Check sheet for the modelled part. Datum: model origin and axes. Units: mm. A direction names the side the tool comes from. Give positions to 0.01 mm unless a question says otherwise; leave off trailing zeros. Order: outer loops, then holes, each group sorted by start corner. A loop starts at its lowest first (then second) coordinate and runs counter-clockwise, first axis right, second up.
from build123d import *

# Parameters (mm, degrees)
SKETCH1_W           = 68
SKETCH1_H           = 68
BOSS_EXTRUDE1_DEPTH = 41
CUT_EXTRUDE1_START  = 41
SKETCH2_W           = 64
SKETCH2_H           = 64
CUT_EXTRUDE1_DEPTH  = 32
CUT_EXTRUDE4_START  = 9
SKETCH3_R           = 23
CUT_EXTRUDE4_DEPTH  = 2
CUT_EXTRUDE9_START  = 7
SKETCH5_R           = 6.05
CUT_EXTRUDE9_DEPTH  = 8
SKETCH6_R           = 10.5
CUT_EXTRUDE10_DEPTH = 5
SKETCH7_W           = 30
SKETCH7_H           = 30
SKETCH7_W_2         = 26
SKETCH7_H_2         = 26
CUT_EXTRUDE11_DEPTH = 2
SKETCH8_R           = 1.5
CUT_EXTRUDE12_DEPTH = 3
SKETCH4_W           = 11
SKETCH4_H           = 16
SKETCH4_R           = 1.75
CUT_EXTRUDE13_DEPTH = 3


with BuildPart() as part:
    # Sketch1 → Boss-Extrude1 (new body)
    with BuildSketch(Plane(origin=(0, 0, 0), x_dir=(1, 0, 0), z_dir=(0, 1, 0))):
        Rectangle(SKETCH1_W, SKETCH1_H)
    extrude(amount=BOSS_EXTRUDE1_DEPTH)

    # Sketch2 → Cut-Extrude1 (cut)
    with BuildSketch(Plane(origin=(0, 0, 0), x_dir=(1, 0, 0), z_dir=(0, 1, 0)).offset(CUT_EXTRUDE1_START)):
        Rectangle(SKETCH2_W, SKETCH2_H)
    extrude(amount=-CUT_EXTRUDE1_DEPTH, mode=Mode.SUBTRACT)

    # Sketch3 → Cut-Extrude4 (cut)
    with BuildSketch(Plane(origin=(0, 0, 0), x_dir=(1, 0, 0), z_dir=(0, 1, 0)).offset(CUT_EXTRUDE4_START)):
        Circle(SKETCH3_R)
    extrude(amount=-CUT_EXTRUDE4_DEPTH, mode=Mode.SUBTRACT)

    # Sketch5 → Cut-Extrude9 (cut, through all)
    with BuildSketch(Plane(origin=(0, 0, 0), x_dir=(1, 0, 0), z_dir=(0, 1, 0)).offset(CUT_EXTRUDE9_START)):
        Circle(SKETCH5_R)
    extrude(amount=-CUT_EXTRUDE9_DEPTH, mode=Mode.SUBTRACT)

    # Sketch6 → Cut-Extrude10 (cut)
    with BuildSketch(Plane.XZ):
        Circle(SKETCH6_R)
    extrude(amount=-CUT_EXTRUDE10_DEPTH, mode=Mode.SUBTRACT)

    # Sketch7 → Cut-Extrude11 (cut)
    with BuildSketch(Plane(origin=(0, 0, 0), x_dir=(-1, 0, 0), z_dir=(0, -1, 0))):
        Rectangle(SKETCH7_W, SKETCH7_H)
        Rectangle(SKETCH7_W_2, SKETCH7_H_2, mode=Mode.SUBTRACT)
    extrude(amount=-CUT_EXTRUDE11_DEPTH, mode=Mode.SUBTRACT)

    # Sketch8 → Cut-Extrude12 (cut, through all)
    with BuildSketch(Plane.ZY.offset(-32)):
        with Locations((-20, 32)):
            Circle(SKETCH8_R)
    extrude(amount=-CUT_EXTRUDE12_DEPTH, mode=Mode.SUBTRACT)

    # Sketch4 → Cut-Extrude13 (cut)
    with BuildSketch(Plane(origin=(0, 7, 0), x_dir=(1, 0, 0), z_dir=(0, 1, 0))):
        with Locations((-18.125903529, 0.086164087)):
            Rectangle(SKETCH4_W, SKETCH4_H)
        with Locations((-16.625903529, 0.086164087)):
            Circle(SKETCH4_R, mode=Mode.SUBTRACT)
    extrude(amount=-CUT_EXTRUDE13_DEPTH, mode=Mode.SUBTRACT)


solid = part.part
1) Section check C-C, the plane y = 32. Record the cut outline in (x, z).
Recorded:
outline: (-34, -34) - (34, -34) - (34, -21.5) - (32, -21.5) - (32, -32) - (-32, -32) - (-32, 32) - (32, 32) - (32, -18.5) - (34, -18.5) - (34, 34) - (-34, 34) - close
2) Depth check by flat-ended pin: pin 1 Ø1.7 at (x, z) = (-22, 3) entering from -Y; pin 2 Ø9 at (x, z) = (-17.5, -2) entering from +Y. Enter the tip coordinate at first touch or a pass-through.
Recorded:
pin 1: stops at y = 0
pin 2: stops at y = 7
3) Draft check along Y on faces 5 (the face through (-18, 6, -8.086)), 6 (the face through (-16, 0, 0)), 7 (the face through (-15, 1, 0)). Enter one of: +Y half, -Y half, draft (parallel to the pull), parting line (faces both ways), or undercut.
Recorded:
face 5: undercut
face 6: -Y half
face 7: draft
4) Section check D-D, the plane x = 29. Record the cut outline in (y, z), then the cut area to 3 significant figures.
Recorded:
outline: (0, -34) - (41, -34) - (41, -32) - (9, -32) - (9, 32) - (41, 32) - (41, 34) - (0, 34) - close
area: 740 mm2
5) Material ranges on L1, parallel to X at y = 5.6, z = 0; L2, parallel to Z at x = 0, y = 1; L3, parallel to X at y = 12, z = -6.5, recorded low to high.
Recorded:
L1: x = -34 to -23.63, -18.37 to -14.88, -12.63 to -6.05, 6.05 to 34
L2: z = -34 to -15, -13 to -10.5, 10.5 to 13, 15 to 34
L3: x = -34 to -32, 32 to 34
6) Section check A-A, the plane x = 0. Record the cut outline in (y, z), then the cut area to 3 significant figures.
Recorded:
outline: (0, -34) - (41, -34) - (41, -32) - (9, -32) - (9, -23) - (7, -23) - (7, -6.05) - (5, -6.05) - (5, -10.5) - (0, -10.5) - (0, -13) - (2, -13) - (2, -15) - (0, -15) - close; (0, 10.5) - (5, 10.5) - (5, 6.05) - (7, 6.05) - (7, 23) - (9, 23) - (9, 32) - (41, 32) - (41, 34) - (0, 34) - (0, 15) - (2, 15) - (2, 13) - (0, 13) - close
area: 511 mm2
7) Set-up check for faces 1 (the face through (-18, 6, 7.914)), 2 (the face through (32.99, 32.07, -21.5)), 3 (the face through (5, 7, 5)), 4 (the face through (13, 1, 0)): record each of +Z, -Z, +X, -X, +Y, -Y from which the full face is reachable in a straight line by a thin tool's end or side.
Recorded:
face 1: none
face 2: +X
face 3: +Y
face 4: -Y
8) Section check B-B, the plane z = 26. Record the cut outline in (x, y).
Recorded:
outline: (-34, 0) - (34, 0) - (34, 41) - (32, 41) - (32, 9) - (-32, 9) - (-32, 41) - (-34, 41) - close
